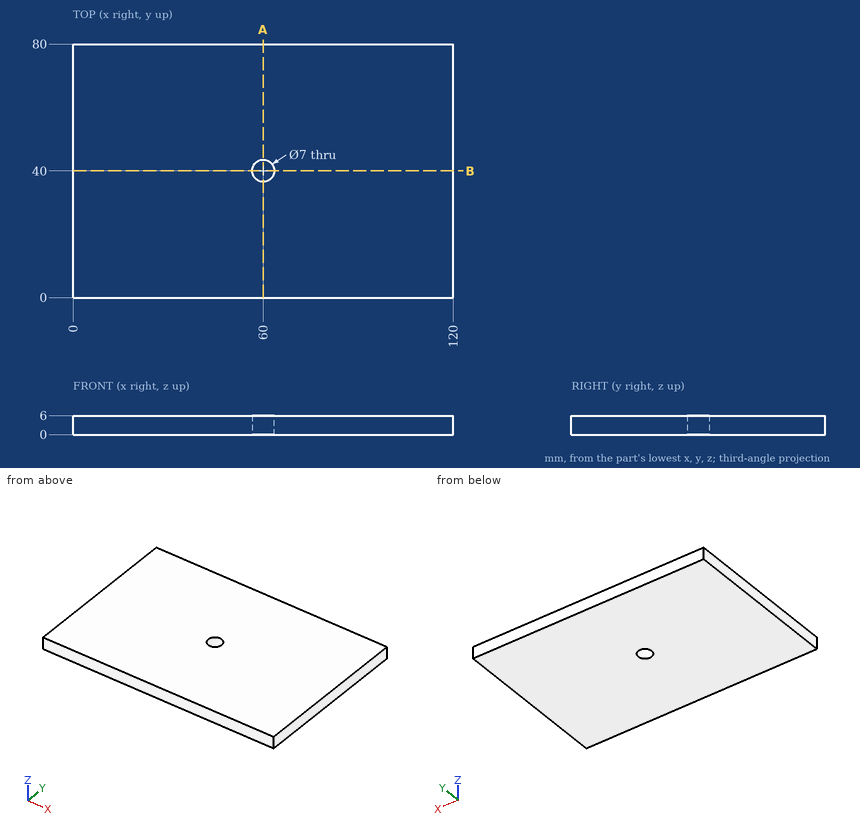
For this review, use the dimensioned drawing (mm, ordinates from the lowest corner) and the shaded views. Coordinates: 2 decimals unless noted, no trailing zeros. Write each loop counter-clockwise with the first axis right and the second up, starting at its lowest first coordinate (ties: lowest second). Pieces come first, ordered by that corner, then holes. Notation, with made-up numbers: (-23, -20.75) - (34, -20.75) arc R7 cw to (34, -14.75) - close; hole circle Ø5 at (-14, -40). An arc over 180 degrees is marked (long way). Answer in a Markdown table with one row per item. Add a question column.
Q1. Consider section B-B on y = 40. Give the boundary of the cut face in (x, z), then the cut area to 3 significant figures.
Q2. To check wall thickness, follow line 1 along Y through (x, z) = (60, 1.85); line 2 along X through (y, z) = (40, 4.25); line 3 along X through (y, z) = (42, 0.6). State the ranges of each line that lie inside material, in increasing order. Write a range as from..to.
Q3. Clearance check with a flat-ended pin moving along its axis: pin 1 (6.5 mm diameter, centred on x = 60, y = 40, fed in from +Z). State where the tip first meets the part, or that it passes through.
Q4. Consider section A-A on x = 60. Give the boundary of the cut face in (y, z), then the cut area to 3 significant figures.
Answers below:
| question | item | result |
|---|---|---|
| 1 | outline | (0, 0) - (56.5, 0) - (56.5, 6) - (0, 6) - close; (63.5, 0) - (120, 0) - (120, 6) - (63.5, 6) - close |
| 1 | area | 678 mm² |
| 2 | line 1 | 0..36.5, 43.5..80 |
| 2 | line 2 | 0..56.5, 63.5..120 |
| 2 | line 3 | 0..57.13, 62.87..120 |
| 3 | pin 1 | through |
| 4 | outline | (0, 0) - (36.5, 0) - (36.5, 6) - (0, 6) - close; (43.5, 0) - (80, 0) - (80, 6) - (43.5, 6) - close |
| 4 | area | 438 mm² |
